```python
from build123d import *

# Parameters (mm, degrees)
SKETCH2_W                  = 33
SKETCH2_H                  = 5
SKETCH3_W                  = 2.217424305
SKETCH3_H                  = 4
CUT_EXTRUDE1_DEPTH         = 41.012498047
M4X0_7_TAPPED_HOLE1_REACH  = 48.446
M4X0_7_TAPPED_HOLE1_BORE_R = 1.65
CIRPATTERN1_COUNT          = 2
CIRPATTERN1_ANGLE          = 90
CHAMFER1_SIZE              = 1
CHAMFER2_SIZE              = 0.5


with BuildPart() as part:
    # Sketch1 → Revolve1 (revolve)
    with BuildSketch(Plane.XY, mode=Mode.PRIVATE) as revolve1_sk:
        Polygon((0, 0), (0, 16), (2, 16), (2, 14.5), (2.5, 14.5), (2.5, 15), (22.5, 15), (22.5, 14.5), (23, 14.5), (23, 16), (25, 16), (25, 12.5), (33, 12.5), (33, 0), align=None)
    revolve(revolve1_sk.sketch.rotate(Axis((-28.053191665, 0, 0), (1, 0, 0)), 90), axis=Axis((-28.053191665, 0, 0), (1, 0, 0)))

    # Sketch2 → Cut-Revolve1 (revolve, cut)
    with BuildSketch(Plane.XY, mode=Mode.PRIVATE) as cut_revolve1_sk:
        with Locations((16.5, 2.5)):
            Rectangle(SKETCH2_W, SKETCH2_H)
    revolve(cut_revolve1_sk.sketch.rotate(Axis((-6.491818973, 0, 0), (1, 0, 0)), 90), axis=Axis((-6.491818973, 0, 0), (1, 0, 0)), mode=Mode.SUBTRACT)

    # Sketch3 → Cut-Extrude1 (cut, through all)
    with BuildSketch(Plane(origin=(33, 0, 0), x_dir=(0, 0, -1), z_dir=(1, 0, 0))):
        with Locations((-5.691287847, 0)):
            Rectangle(SKETCH3_W, SKETCH3_H)
    extrude(amount=-CUT_EXTRUDE1_DEPTH, mode=Mode.SUBTRACT)

    # M4x0.7 Tapped Hole1 bore → M4x0.7 Tapped Hole1 (cut, up to next)
    with BuildSketch(Plane.XY.offset(12.5), mode=Mode.PRIVATE) as m4x0_7_tapped_hole1_sk1:
        with Locations((29, 0)):
            Circle(M4X0_7_TAPPED_HOLE1_BORE_R)
    m4x0_7_tapped_hole1_tool1 = extrude(m4x0_7_tapped_hole1_sk1.sketch, amount=-M4X0_7_TAPPED_HOLE1_REACH, mode=Mode.PRIVATE) & part.part
    m4x0_7_tapped_hole1 = m4x0_7_tapped_hole1_tool1.solids().sort_by_distance((29, 0, 12.5))[0]
    add(m4x0_7_tapped_hole1, mode=Mode.SUBTRACT)

    # CirPattern1: M4x0.7 Tapped Hole1; each copy of M4x0.7 Tapped Hole1 runs up to whatever stops it at its own place
    cirpattern1_before = part.part  # the part as the pattern finds it: every copy runs up to it
    cirpattern1_m4x0_7_tapped_hole1_long = extrude(m4x0_7_tapped_hole1_sk1.sketch, amount=-M4X0_7_TAPPED_HOLE1_REACH, mode=Mode.PRIVATE)
    cirpattern1_m4x0_7_tapped_hole1_tool1 = cirpattern1_m4x0_7_tapped_hole1_long.rotate(Axis((-6.491818973, 0, 0), (1, 0, 0)), 1 * CIRPATTERN1_ANGLE / (CIRPATTERN1_COUNT - 1)) & cirpattern1_before
    add(cirpattern1_m4x0_7_tapped_hole1_tool1.solids().sort_by_distance((29, -12.5, 0))[0], mode=Mode.SUBTRACT)

    # Chamfer1
    chamfer1_edges = [part.edges().sort_by_distance(p)[0] for p in [
        (33, 0, -12.5),
    ]]
    chamfer(chamfer1_edges, length=CHAMFER1_SIZE)

    # Chamfer2
    chamfer2_edges = [part.edges().sort_by_distance(p)[0] for p in [
        (25, 0, -16),
        (0, 0, -16),
    ]]
    chamfer(chamfer2_edges, length=CHAMFER2_SIZE)


solid = part.part
```
Could you check a few things on this model? Use its own coordinates, in mm. A direction names the side the tool comes from. Round coordinates to 2 decimals unless told otherwise and drop trailing zeros. Loops run counter-clockwise (first coordinate to the right, second up) from the corner with the lowest first, then second, coordinate; pieces in that order, holes last. Notation, with made-up numbers: (39.25, -17.5) - (44.25, -17.5) arc R22 cw to (44.25, -3.5) - close; hole circle Ø6 at (61.25, 20.5). An arc over 180 degrees is marked (long way). Answer in a Markdown table with one row per item. Add a question column.
(1) If we mould it in two halves opening along X, with no side actions, what happens to faces 5 (the face through (25, -13, 1)), 6 (the face through (27.35, 0.07, 9.69)), 7 (the face through (17, 2, 6)), 8 (the face through (0, -4, 4))? For each: pulls with the +X half, pulls with the -X half, needs draft (parallel to the pull), parting line crosses it, or undercut.
(2) I need wall thicknesses on line 1 along X through (y, z) = (8.5, -12); line 2 along X through (y, z) = (0, 10); line 3 along Y through (x, z) = (26.5, 0). Which ranges of each line are inside material? Lowest first, please.
(3) If we section it at B-B (z = 0): State how many separate pieces and enclosed holes the cut face has, plus the area to 3 significant figures.
(4) For faces 1 (the face through (17, -2, 6)), 2 (the face through (27.69, -8.66, -1)), 3 (the face through (33, 2.4, 5)), 4 (the face through (22.754, 12.864, 6.691)), which set-ups out of +Z, -Z, +X, -X, +Y, -Y let a thin tool reach every point of the face, with its end or its side?
(5) If we section it at C-C (x = 29): Please give me the cut outline in (y, z), plus the area to 3 significant figures.
(6) If we section it at A-A (x = 17): Please give me the cut outline in (y, z).
(7) I'm going to push flat-ended pins straight in: pin 1 (4 mm diameter, centred on x = 9, z = -12.5, fed in from +Y); pin 2 (3 mm diameter, centred on x = 21, y = -0.5, fed in from -Z); pin 3 (2 mm diameter, centred on x = 29, y = 0, fed in from -Z); pin 4 (16 mm diameter, centred on y = -7, z = -4, fed in from -X). Where does each tip first touch, or does it pass through?
Model answer:
| question | item | result |
|---|---|---|
| 1 | face 5 | pulls with the +X half |
| 1 | face 6 | undercut |
| 1 | face 7 | needs draft |
| 1 | face 8 | pulls with the -X half |
| 2 | line 1 | x = 0 to 2, 2.5 to 22.5, 23 to 25 |
| 2 | line 2 | x = 0 to 27.35, 30.65 to 33 |
| 2 | line 3 | y = -12.5 to -5, 5 to 12.5 |
| 3 | separate pieces | 3 |
| 3 | enclosed holes | 0 |
| 3 | area | 601 mm² |
| 4 | face 1 | +X, -X |
| 4 | face 2 | -Y |
| 4 | face 3 | +Z, -Z, +X, +Y, -Y |
| 4 | face 4 | none |
| 5 | outline | (-12.39, -1.65) arc R12.5 ccw (long way) to (1.65, 12.39) - (1.65, 6.8) - (2, 6.8) - (2, 4.58) arc R5 cw (long way) to (-4.72, -1.65) - close; (-12.39, 1.65) - (-4.72, 1.65) arc R5 cw to (-2, 4.58) - (-2, 6.8) - (-1.65, 6.8) - (-1.65, 12.39) arc R12.5 ccw to start |
| 5 | area | 361 mm² |
| 6 | outline | circle Ø30 at (0, 0); hole (-2, 4.58) arc R5 ccw (long way) to (2, 4.58) - (2, 6.8) - (-2, 6.8) - close |
| 7 | pin 1 | stops at y = 10.71 |
| 7 | pin 2 | stops at z = -15 |
| 7 | pin 3 | stops at z = -12.5 |
| 7 | pin 4 | stops at x = 0 |
